Geometry check sheet. Reference: drawing and pictorial views, mm from the part's lowest x, y, z. A direction names the side the tool comes from. Give positions to 0.01 mm unless a question says otherwise; leave off trailing zeros. Write each loop counter-clockwise with the first axis right and the second up, starting at its lowest first coordinate (ties: lowest second). Pieces come first, ordered by that corner, then holes. Notation, with made-up numbers: (43, 73) - (70, 73) arc R22 ccw to (70, 80) - close; hole circle Ø6 at (40, 55). An arc over 180 degrees is marked (long way). Write item = value, one per line. Start each with the question number.
(1) Section check A-A, the plane z = 19. Enter the section's corners in (x, y), plus the area to 3 significant figures.
(2) Access from +Z, -Z, +X, -X, +Y, -Y to the whole of each face (thin tool, end or side, straight path). Record for the marked faces 1 and 2.
(3) Depth check by flat-ended pin: pin 1 Ø2.5 at (x, y) = (3, 3) entering from -Z; pin 2 Ø1 at (x, z) = (4, 38) entering from +Y; pin 3 Ø2 at (x, z) = (4.5, 36) entering from -Y. Enter the tip coordinate at first touch or a pass-through.
(4) Thickness scan on L1, parallel to X at y = 0.8, z = 10; L2, parallel to Y at x = 2.4, z = 26.5; L3, parallel to Y at x = 4.05, z = 37.5. Record the ranges inside material, lowest first.
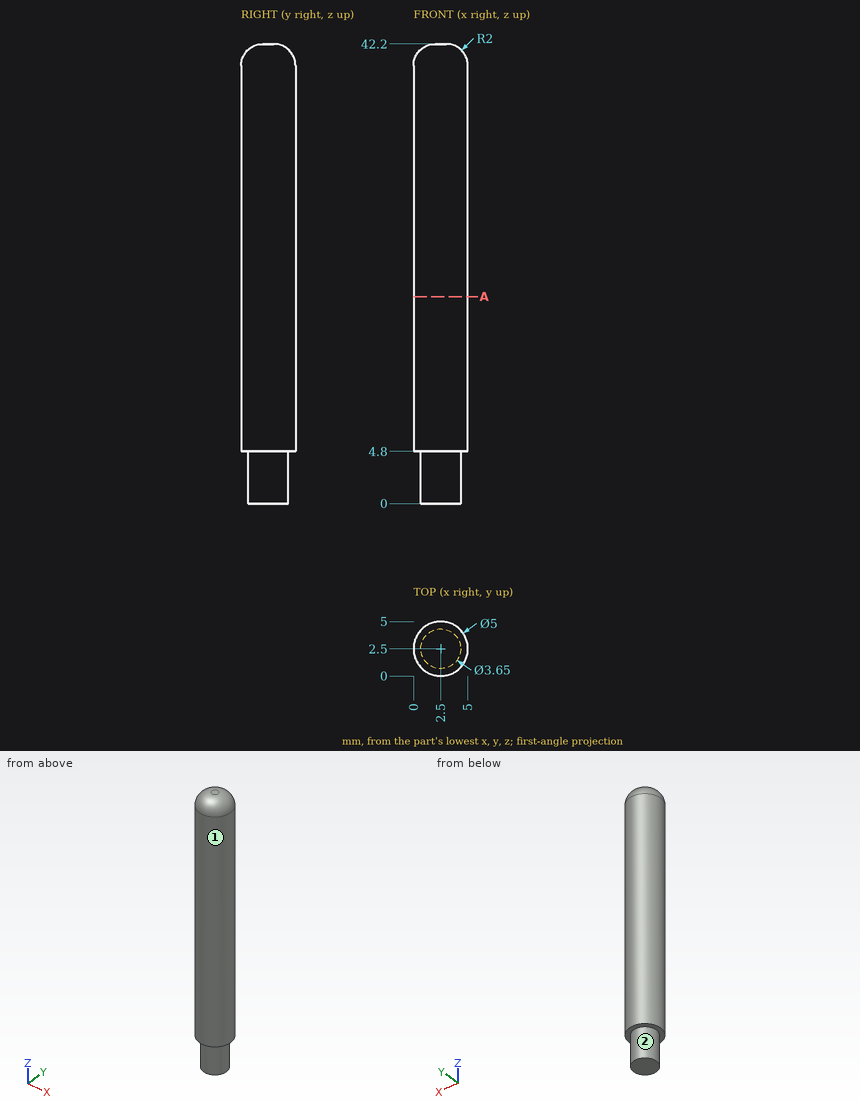
Model answer:
q1.outline = circle Ø5 at (2.5, 2.5)
q1.area = 19.6 mm²
q2.face_1 = +Z, -Z
q2.face_2 = -Z
q3.pin_1 = 0
q3.pin_2 = 4.79
q3.pin_3 = 0.21
q4.L1 = 0.67 to 4.33
q4.L2 = 0 to 5
q4.L3 = 0.54 to 4.46
